Input: part model. Units: mm. Frame: model coordinates. Face numbers are marked on the shaded views. A direction names the side the tool comes from. Give positions to 0.01 mm unless a question says otherwise; leave off trailing zeros. Loops run counter-clockwise (first coordinate to the right, second up) from the corner with the lowest first, then second, coordinate; pieces in that order, holes last. Notation, with made-up numbers: M -13.5,10.25 L 32.5,10.25 A27 ccw 32.5,43.25 Z; hole C 77.25,1.5 d7. An arc over 180 degrees is marked long. Answer as a JSON object with one key per item and string values. Group by question number.
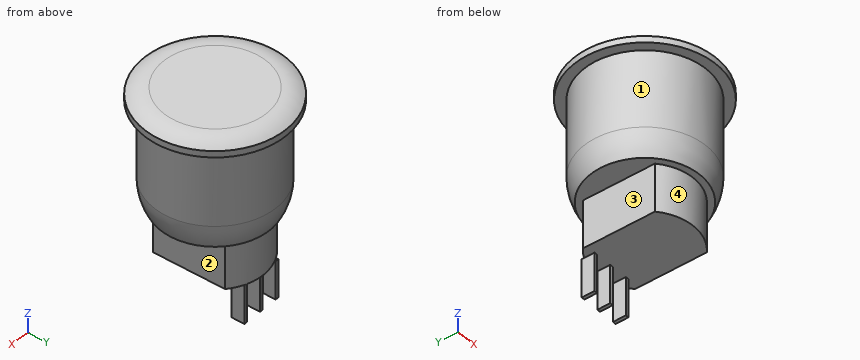
Autodesk Inventor part; units mm, degrees
ref_plane "YZ Plane" through (0, 0, 0) normal (1, 0, 0) x (0, 1, 0)
ref_plane "XZ Plane" through (0, 0, 0) normal (0, 1, 0) x (-1, 0, 0)
ref_plane "XY Plane" through (0, 0, 0) normal (0, 0, 1) x (1, 0, 0)
sketch "Skizze1" plane through (0, 0, 0) normal (0, 1, 0) x (-1, 0, 0)
  line L0 (0, 0) -> (0, -100) construction
  line L1 (0, 0) -> (8, 0)
  arc A0 (11, -1) -> (8, 0) centre (8, -5) ccw
  line L2 (11, -1) -> (11, -2)
  line L3 (11, -2) -> (9.5, -2)
  line L4 (9.5, -2) -> (9.5, -14)
  arc A1 (8.5, -18) -> (9.5, -14) centre (1, -14) ccw
  line L5 (8.5, -18) -> (7.5, -18)
  line L6 (7.5, -18) -> (7.5, -25.5)
  line L7 (7.5, -25.5) -> (0, -25.5)
  line L8 (0, 0) -> (0, -25.5)
  point P0 (10.25, -2)
  dimension "d0" = 100
  dimension "d1" = 19
  dimension "d2" = 22
  dimension "d3" = 2
  dimension "d4" = 1
  dimension "d5" = 3
  dimension "d6" = 12
  dimension "d7" = 4
  dimension "d10" = 7.5
  dimension "d26" = 7.5
  dimension "d27" = 8.5
revolve "Umdrehung1" add sketch "Skizze1" angle 360 about axis through (0, 0, 0) along (0, 0, -1)
thread "Gewinde1"
sketch "Skizze2" plane through (0, 0, -25.5) normal (0, 0, -1) x (-1, 0, 0)
  circle A0 centre (0, 0) radius 7.5
  line L0 (5, 5.5902) -> (-5, 5.5902)
  line L1 (-5, 5.5902) -> (-5, -5.5902)
  line L2 (-5, -5.5902) -> (5, -5.5902)
  line L3 (5, -5.5902) -> (5, 5.5902)
  point P0 (-5, 5.5902)
  dimension "d14" = 10
extrude "Extrusion1" cut sketch "Skizze2" against normal up to surface (7.5 mm away) contours A0 L3 | L1 A0
sketch "Skizze3" plane through (0, 0, -25.5) normal (0, 0, -1) x (-1, 0, 0)
  line L0 (3.5, 7) -> (3, 7)
  line L1 (3, 7) -> (3, 5)
  line L2 (3, 5) -> (3.5, 5)
  line L3 (3.5, 5) -> (3.5, 7)
  point P0 (0, 0)
  point P1 (3, 6)
  dimension "d17" = 0.5
  dimension "d18" = 2
  dimension "d19" = 5
  dimension "d20" = 3
extrude "Extrusion2" add sketch "Skizze3" along normal blind 6
pattern_linear "Rechteckige Anordnung1" count 3 spacing 3 along (1, 0, 0) of "Extrusion2"
properties part number "Druckknopf_Konsole_groß" material "Stahl, galvanisiert"
1. First-contact query: P1, Ø3, axis at x = 1.5, y = 0.5, coming from the -Z side; P2, Ø12, axis at x = 5, z = -16.5, coming from the +Y side; P3, Ø2, axis at x = -2, z = -8.5, coming from the -Y side; P4, Ø1.5, axis at x = 2, y = 3, coming from the +Z side. Flat tips, straight axial feed; report the tip coordinate or a pass-through.
2. Reachability of the marked faces 1, 2, 3 and 4 from +Z, -Z, +X, -X, +Y, -Y: full face, straight path, thin tool, end or side. Return the list, or none.
3. Section A-A (z = -12). Output: boundary loops of the cut face in (x, y).
4. Material intervals for L1, parallel to X at y = 4.25, z = -22; L2, parallel to Z at x = -2.5, y = 5; L3, parallel to Y at x = -4.25, z = -5, sorted ascending.
Geometry results:
{
 "1": {"P1": "z = -25.5", "P2": "y = 9.5", "P3": "y = -9.45", "P4": "z = 0"},
 "2": {"face 1": "-Z", "face 2": "-Z, +X, +Y, -Y", "face 3": "-Z, -X, +Y, -Y", "face 4": "-Z, -Y"},
 "3": {"outline": "C 0,0 d19"},
 "4": {"L1": "-5 to 5", "L2": "-25.5 to 0", "L3": "-8.5 to 8.5"}
}
